Verification items for this drawing (mm, ordinates from the low corner). A direction names the side the tool comes from. Coordinates: 2 decimals unless noted, no trailing zeros. Order: outer loops, then holes, each group sorted by start corner. A loop starts at its lowest first (then second) coordinate and runs counter-clockwise, first axis right, second up. Notation, with made-up numbers: (75, -15) - (101, -15) arc R16 ccw to (101, -10) - close; hole circle Ø6 at (28.25, 60). An arc over 180 degrees is marked (long way). Use CSV: the item, a comma, the result in double quotes. Start each with the question number.
1) Sectioned sample at C-C, the plane y = 36.9. Record the cut outline in (x, z).
2) Sectioned sample at D-D, the plane x = 20. Record the cut outline in (y, z) (1 decimal).
3) Sectioned sample at B-B, the plane x = 31.9. Record the cut outline in (y, z).
4) Sectioned sample at A-A, the plane z = 31. Count the separate pieces of the cut face and the enclosed holes in it, and give its area (3 significant figures).
5) Thickness scan on probe 1 along X at (y, z) = (60, 33) (1 decimal); probe 2 along Y at (x, z) = (31, 35) (1 decimal); probe 3 along Y at (x, z) = (56, 8) (1 decimal). Record the ranges inside material, lowest first. Write a range as [from, to].
6) Tool access check on the marked faces 4 and 5. Record the directions out of +Z, -Z, +X, -X, +Y, -Y that give a thin tool (end or side, any length) a straight path to the whole face; none if there is none.
7) Draft check along Y on the marked faces 1, 2 and 3. Enter one of: released by +Y, released by -Y, zero draft, split by the parting line, or undercut.
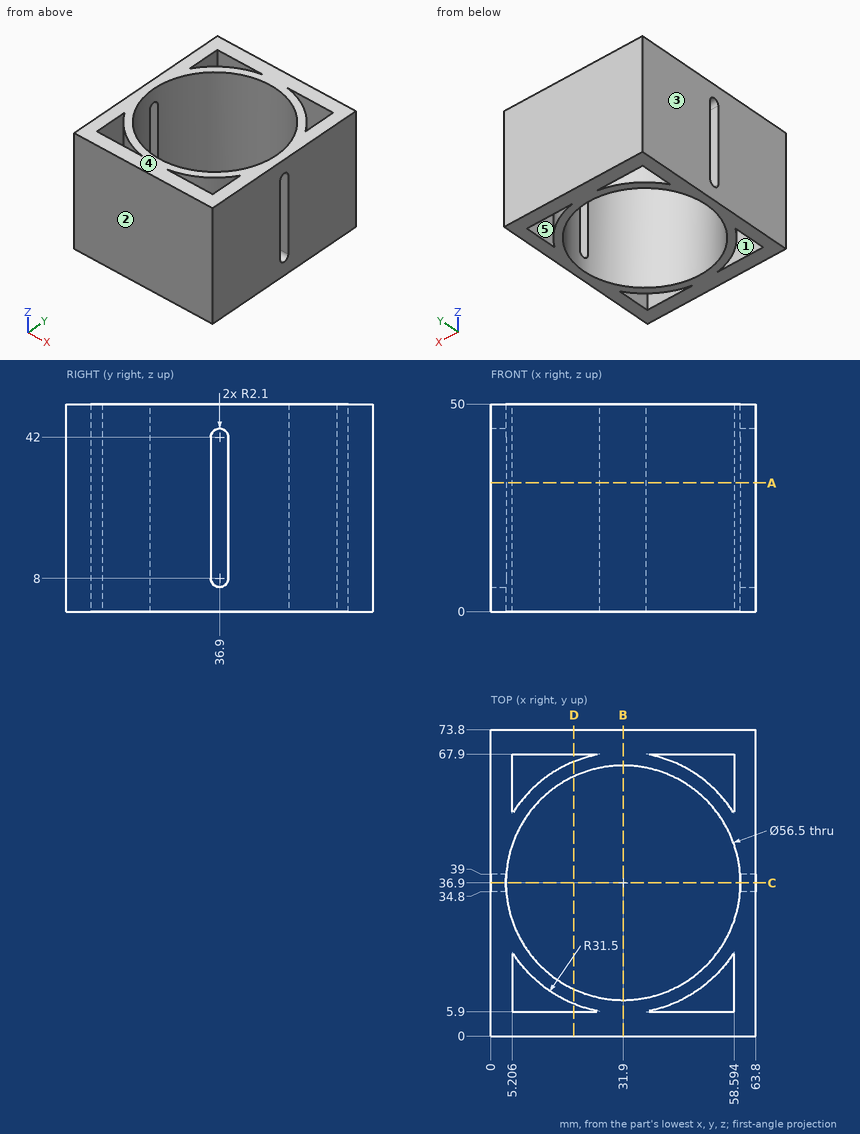
Evaluation:
1,outline,"(0, 0) - (3.65, 0) - (3.65, 5.9) - (0, 5.9) - close; (0, 44.1) - (3.65, 44.1) - (3.65, 50) - (0, 50) - close; (60.15, 0) - (63.8, 0) - (63.8, 5.9) - (60.15, 5.9) - close; (60.15, 44.1) - (63.8, 44.1) - (63.8, 50) - (60.15, 50) - close"
2,outline,"(0, 0) - (5.9, 0) - (5.9, 50) - (0, 50) - close; (7.7, 0) - (11.3, 0) - (11.3, 50) - (7.7, 50) - close; (62.5, 0) - (66.1, 0) - (66.1, 50) - (62.5, 50) - close; (67.9, 0) - (73.8, 0) - (73.8, 50) - (67.9, 50) - close"
3,outline,"(0, 0) - (8.65, 0) - (8.65, 50) - (0, 50) - close; (65.15, 0) - (73.8, 0) - (73.8, 50) - (65.15, 50) - close"
4,separate pieces,"2"
4,enclosed holes,"4"
4,area,"1,750 mm²"
5,probe 1,"[0, 5.2], [10.5, 15.6], [48.2, 53.3], [58.6, 63.8]"
5,probe 2,"[0, 8.7], [65.1, 73.8]"
5,probe 3,"[0, 5.9], [16.6, 22.2], [51.6, 57.2], [67.9, 73.8]"
6,face 4,"+Z, +X, -X, +Y, -Y"
6,face 5,"+Z, -Z"
7,face 1,"undercut"
7,face 2,"released by -Y"
7,face 3,"zero draft"
